Build history of the part. All positions in model axes, mm. A direction names the side the tool comes from. Give positions to 0.01 mm unless a question says otherwise; leave off trailing zeros. Order: outer loops, then holes, each group sorted by start corner. A loop starts at its lowest first (then second) coordinate and runs counter-clockwise, first axis right, second up. Notation, with made-up numbers: (8, 75.25) - (30, 75.25) arc R14 cw to (30, 96.25) - close; hole circle Ø10 at (9.25, 15.25). An arc over 180 degrees is marked (long way). Write each question's results on one line, items separated by ' | '. Start each with the question number.
1) Tool access for faces 4 (the face through (-1, 30.48, 15)), 5 (the face through (-2.54, 15, 1)), 6 (the face through (0, 15, 1)): list every direction of +Z, -Z, +X, -X, +Y, -Y with a clear straight run to the whole face (end or side of a thin tool).
2) Drill centre lines: line 1 along Z through (x, y) = (0.25, 33); line 2 along X through (y, z) = (38, 4); line 3 along X through (y, z) = (20, 26). Where is each one in solid material? Low to high. Write a range as from..to.
3) Two-plate mould, pull along Y, no slides. Class faces 1 (the face through (-3, 36, -22.86)), 2 (the face through (-1, 0, 0)), 3 (the face through (-0.69, 35, -0.11)): +Y half, -Y half, draft (parallel to the pull), parting line (faces both ways), or undercut.
4) Cut at D-D on x = 4.75. List the corners of the cut face in (y, z), plus the area to 3 significant figures.
5) Cut at C-C on x = -1.25. List the corners of the cut face in (y, z).
6) Cut at A-A on y = 38.1. List the corners of the cut face in (x, z) (3 decimals).
7) Drop flat-ended pins along their axis: pin 1 Ø2 at (x, z) = (-1.5, 13.5) entering from +Y; pin 2 Ø5 at (x, z) = (-4, 2) entering from -Y; pin 3 Ø4 at (y, z) = (10, 3) entering from +X; pin 4 Ø3 at (y, z) = (18, 11) entering from -X. Give the stop position or say it passes through.
from build123d import *

# Parameters (mm, degrees)
SKETCH1_R           = 5.715
SKETCH1_R_2         = 3.175
BOSS_EXTRUDE1_DEPTH = 38.1
SKETCH2_R           = 3.175
CUT_EXTRUDE1_DEPTH  = 7.62
FILLET1_R           = 2.54


with BuildPart() as part:
    # Sketch1 → Boss-Extrude1 (new body, symmetric)
    with BuildSketch(Plane.XY):
        with BuildLine():
            Line((-2.54, 0), (0, 0))
            Line((0, 0), (0, 30.48))
            ThreePointArc((0, 30.48), (-0.096177955, 31.457600747), (-0.381023909, 32.39771574))
            ThreePointArc((-0.381023909, 32.39771574), (-2.351034724, 32.890982749), (-4.024171598, 34.042011834))
            ThreePointArc((-4.024171598, 34.042011834), (-2.925884615, 32.409423077), (-2.54, 30.48))
            Line((-2.54, 30.48), (-2.54, 0))
        make_face()
        with Locations((0, 38.1)):
            Circle(SKETCH1_R)
        with Locations((0, 38.1)):
            Circle(SKETCH1_R_2, mode=Mode.SUBTRACT)
    extrude(amount=BOSS_EXTRUDE1_DEPTH, both=True)

    # Sketch2 → Cut-Extrude1 (cut, symmetric)
    with BuildSketch(Plane.XY.offset(15.24)):
        with BuildLine():
            ThreePointArc((0, 30.48), (-0.096177955, 31.457600747), (-0.381023909, 32.39771574))
            ThreePointArc((-0.381023909, 32.39771574), (2.351034724, 43.309017251), (-4.024171598, 34.042011834))
            ThreePointArc((-4.024171598, 34.042011834), (-2.925884615, 32.409423077), (-2.54, 30.48))
            Line((-2.54, 30.48), (0, 30.48))
        make_face()
        with Locations((0, 38.1)):
            Circle(SKETCH2_R, mode=Mode.SUBTRACT)
    cut_extrude1 = extrude(amount=CUT_EXTRUDE1_DEPTH, both=True, mode=Mode.SUBTRACT)

    # Mirror1: Cut-Extrude1 across plane
    add(cut_extrude1.mirror(Plane.XY), mode=Mode.SUBTRACT)

    # Fillet1
    fillet1_edges = [part.edges().sort_by_distance(p)[0] for p in [
        (-1.27, 0, 38.1),
        (-1.27, 0, -38.1),
    ]]
    fillet(fillet1_edges, radius=FILLET1_R)


solid = part.part
Results:
1) face 4: +X, -X, +Y | face 5: +Z, -Z, -X, -Y | face 6: +Z, -Z, +X, -Y
2) line 1: -38.1..-22.86, -7.62..7.62, 22.86..38.1 | line 2: -5.71..-3.17, 3.17..5.71 | line 3: -2.54..0
3) face 1: draft | face 2: -Y half | face 3: undercut
4) outline: (34.92, -38.1) - (41.28, -38.1) - (41.28, -22.86) - (34.92, -22.86) - close; (34.92, -7.62) - (41.28, -7.62) - (41.28, 7.62) - (34.92, 7.62) - close; (34.92, 22.86) - (41.28, 22.86) - (41.28, 38.1) - (34.92, 38.1) - close | area: 291 mm^2
5) outline: (0, -35.56) arc R2.54 ccw to (2.54, -38.1) - (35.18, -38.1) - (35.18, -22.86) - (30.48, -22.86) - (30.48, -7.62) - (35.18, -7.62) - (35.18, 7.62) - (30.48, 7.62) - (30.48, 22.86) - (35.18, 22.86) - (35.18, 38.1) - (2.54, 38.1) arc R2.54 ccw to (0, 35.56) - close; (41.02, -38.1) - (43.68, -38.1) - (43.68, -22.86) - (41.02, -22.86) - close; (41.02, -7.62) - (43.68, -7.62) - (43.68, 7.62) - (41.02, 7.62) - close; (41.02, 22.86) - (43.68, 22.86) - (43.68, 38.1) - (41.02, 38.1) - close
6) outline: (-5.715, -38.1) - (-3.175, -38.1) - (-3.175, -22.86) - (-5.715, -22.86) - close; (-5.715, -7.62) - (-3.175, -7.62) - (-3.175, 7.62) - (-5.715, 7.62) - close; (-5.715, 22.86) - (-3.175, 22.86) - (-3.175, 38.1) - (-5.715, 38.1) - close; (3.175, -38.1) - (5.715, -38.1) - (5.715, -22.86) - (3.175, -22.86) - close; (3.175, -7.62) - (5.715, -7.62) - (5.715, 7.62) - (3.175, 7.62) - close; (3.175, 22.86) - (5.715, 22.86) - (5.715, 38.1) - (3.175, 38.1) - close
7) pin 1: y = 30.48 | pin 2: y = 0 | pin 3: x = 0 | pin 4: x = -2.54
